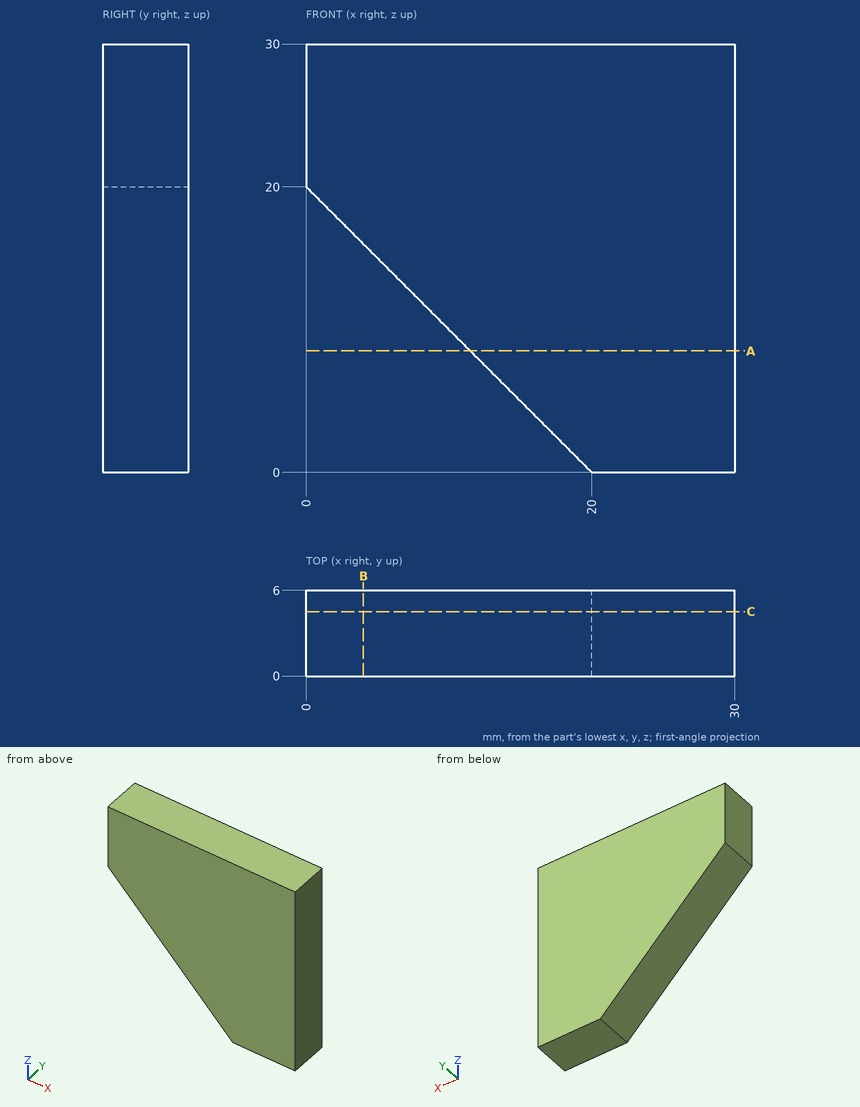
Answer from the drawing. Dimensions are ordinates in mm from the lowest x, y and z of the part. Coordinates: 2 decimals unless noted, no trailing zeros. Order: outer loops, then holes, each group sorted by start corner. A loop starts at its lowest first (then second) coordinate and runs counter-clockwise, first axis right, second up. Notation, with made-up numbers: (8, 52) - (58, 52) arc R22 cw to (58, 91) - close; hole circle Ø1 at (17, -4). An arc over 180 degrees is marked (long way). Answer as a JSON object with one key per item and string values. Group by question number.
Item 1: Section C-C (y = 4.5) is taken. Give the vertices of the cut face in (x, z).
Item 2: A flat-ended cylindrical pin translates along its axis: P1, Ø1.5, axis at x = 17.5, y = 4.5, coming from the -Z side. Find the tip coordinate at first contact, or state that the pin passes through.
Item 3: Consider probe 1 along Z at (x, y) = (12.75, 1); probe 2 along X at (y, z) = (1.75, 7.75); probe 3 along X at (y, z) = (0.75, 17.25). Determine where each line is inside the solid, lowest interval first. Write a range as from..to.
Item 4: Section A-A (z = 8.5) is taken. Give the vertices of the cut face in (x, y), plus the area to 3 significant figures.
Item 5: Section B-B (x = 4) is taken. Give the vertices of the cut face in (y, z), plus the area to 3 significant figures.
Results are:
{
 "1": {"outline": "(0, 20) - (20, 0) - (30, 0) - (30, 30) - (0, 30) - close"},
 "2": {"P1": "stops at z = 1.75"},
 "3": {"probe 1": "z = 7.25..30", "probe 2": "x = 12.25..30", "probe 3": "x = 2.75..30"},
 "4": {"outline": "(11.5, 0) - (30, 0) - (30, 6) - (11.5, 6) - close", "area": "111 mm^2"},
 "5": {"outline": "(0, 16) - (6, 16) - (6, 30) - (0, 30) - close", "area": "84.0 mm^2"}
}
